Verification items for the finished model (mm, model axes). Coordinates: 2 decimals unless noted, no trailing zeros. Write each loop counter-clockwise with the first axis right and the second up, starting at its lowest first coordinate (ties: lowest second). Pieces come first, ordered by that corner, then holes. Notation, with made-up numbers: (-37.75, 52.25) - (5.25, 52.25) arc R18 cw to (5.25, 58.25) - close; hole circle Ø5 at (-34, 10). An arc over 180 degrees is marked (long way). Use one line per item in the form item = value. Start each with the question number.
(1) Sectioned sample at D-D (y = -33). Record the cut outline in (x, z).
(2) Sectioned sample at B-B (z = 1.95). Count the separate pieces of the cut face and the enclosed holes in it, and give its area (3 significant figures).
(3) Material ranges on line 1 (Y direction, x = 0, z = 2.3); line 2 (X direction, y = 97.5, z = 1.65), recorded low to high. Write a range as [from, to].
(4) Sectioned sample at A-A (x = 0). Record the cut outline in (y, z), and give its area (3 significant figures).
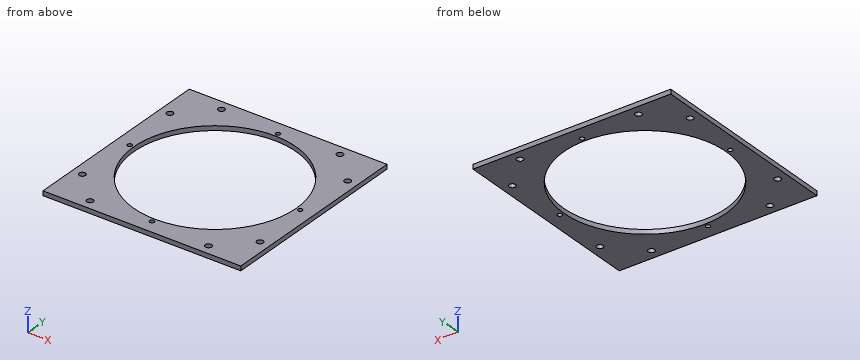
from build123d import *

# Parameters (mm, degrees)
SKETCH2_W           = 217
SKETCH2_H           = 217
SKETCH2_R           = 89
SKETCH2_R_2         = 3.5
BOSS_EXTRUDE1_DEPTH = 5
M6_TAPPED_HOLE1_D   = 5
CIRPATTERN1_COUNT   = 4


with BuildPart() as part:
    # Sketch2 → Boss-Extrude1 (new body)
    with BuildSketch(Plane.XY):
        Rectangle(SKETCH2_W, SKETCH2_H)
        Circle(SKETCH2_R, mode=Mode.SUBTRACT)
        with Locations((-97.5, -65)):
            Circle(SKETCH2_R_2, mode=Mode.SUBTRACT)
        with Locations((-97.5, 65)):
            Circle(SKETCH2_R_2, mode=Mode.SUBTRACT)
        with Locations(Location((97.5, 65, 0), (0, 0, 180))):
            Circle(SKETCH2_R_2, mode=Mode.SUBTRACT)
        with Locations(Location((97.5, -65, 0), (0, 0, 180))):
            Circle(SKETCH2_R_2, mode=Mode.SUBTRACT)
        with Locations((-65, -97.5)):
            Circle(SKETCH2_R_2, mode=Mode.SUBTRACT)
        with Locations((65, -97.5)):
            Circle(SKETCH2_R_2, mode=Mode.SUBTRACT)
        with Locations(Location((65, 97.5, 0), (0, 0, 180))):
            Circle(SKETCH2_R_2, mode=Mode.SUBTRACT)
        with Locations(Location((-65, 97.5, 0), (0, 0, 180))):
            Circle(SKETCH2_R_2, mode=Mode.SUBTRACT)
    extrude(amount=BOSS_EXTRUDE1_DEPTH)

    # M6 Tapped Hole1 (through all)
    with Locations(Plane(origin=(0, 0, 0), x_dir=(-1, 0, 0), z_dir=(0, 0, -1))):
        with Locations((0, -93.5)):
            m6_tapped_hole1 = Hole(M6_TAPPED_HOLE1_D / 2)

    # CirPattern1: M6 Tapped Hole1 ×4 about axis
    cirpattern1_axis = Axis((0, 0, 0), (0, 0, 1))
    for i in range(1, CIRPATTERN1_COUNT):
        add(m6_tapped_hole1.rotate(cirpattern1_axis, i * 360 / CIRPATTERN1_COUNT), mode=Mode.SUBTRACT)


solid = part.part
Answers below:
q1.outline = (-108.5, 0) - (-82.66, 0) - (-82.66, 5) - (-108.5, 5) - close; (82.66, 0) - (108.5, 0) - (108.5, 5) - (82.66, 5) - close
q2.separate_pieces = 1
q2.enclosed_holes = 13
q2.area = 21,800 mm2
q3.line_1 = [-108.5, -96], [-91, -89], [89, 91], [96, 108.5]
q3.line_2 = [-108.5, -68.5], [-61.5, 61.5], [68.5, 108.5]
q4.outline = (-108.5, 0) - (-96, 0) - (-96, 5) - (-108.5, 5) - close; (-91, 0) - (-89, 0) - (-89, 5) - (-91, 5) - close; (89, 0) - (91, 0) - (91, 5) - (89, 5) - close; (96, 0) - (108.5, 0) - (108.5, 5) - (96, 5) - close
q4.area = 145 mm2
